Source: three-view drawing plus pictorial views. Frame: mm from the lowest corner of the part. A direction names the side the tool comes from. Coordinates: 2 decimals unless noted, no trailing zeros. Loops run counter-clockwise (first coordinate to the right, second up) from the corner with the lowest first, then second, coordinate; pieces in that order, holes last. Notation, with made-up numbers: M -2.75,83 L 10.25,83 A20 ccw 10.25,114 Z; hole C 43.5,-23 d9. An arc over 180 degrees is marked long. Use a Markdown table: item, result. Add a question column.
1. Set-up query: the marked faces 4 and 5. Return all of +Z, -Z, +X, -X, +Y, -Y with unobstructed straight access to the full face (end or side cutting, diameter ignored); none if empty.
2. Pin query (flat end, axial travel): pin 1 (4.5 mm diameter, centred on y = 13, z = 6.5, fed in from +X); pin 2 (3 mm diameter, centred on x = 29.95, y = 8, fed in from +Z); pin 3 (1.3 mm diameter, centred on y = 3, z = 8, fed in from +X). Return the tip coordinate at first contact, or that it passes through.
3. Section C-C on z = 20. Output: boundary loops of the cut face in (x, y).
4. Line query: L1, parallel to Y at x = 0.95, z = 7.5; L2, parallel to Z at x = 12, y = 10.75; L3, parallel to X at y = 9.75, z = 6.5. Output: solid intervals per line, ascending. Write a range as [from, to].
5. Draft query along Z for the marked faces 1, 2 and 3. Return one class per face: +Z half, -Z half, draft (parallel to the pull), parting line (faces both ways), or undercut.
6. Section B-B on y = 8. Output: boundary loops of the cut face in (x, z).
7. Section A-A on x = 6.5. Output: boundary loops of the cut face in (y, z).
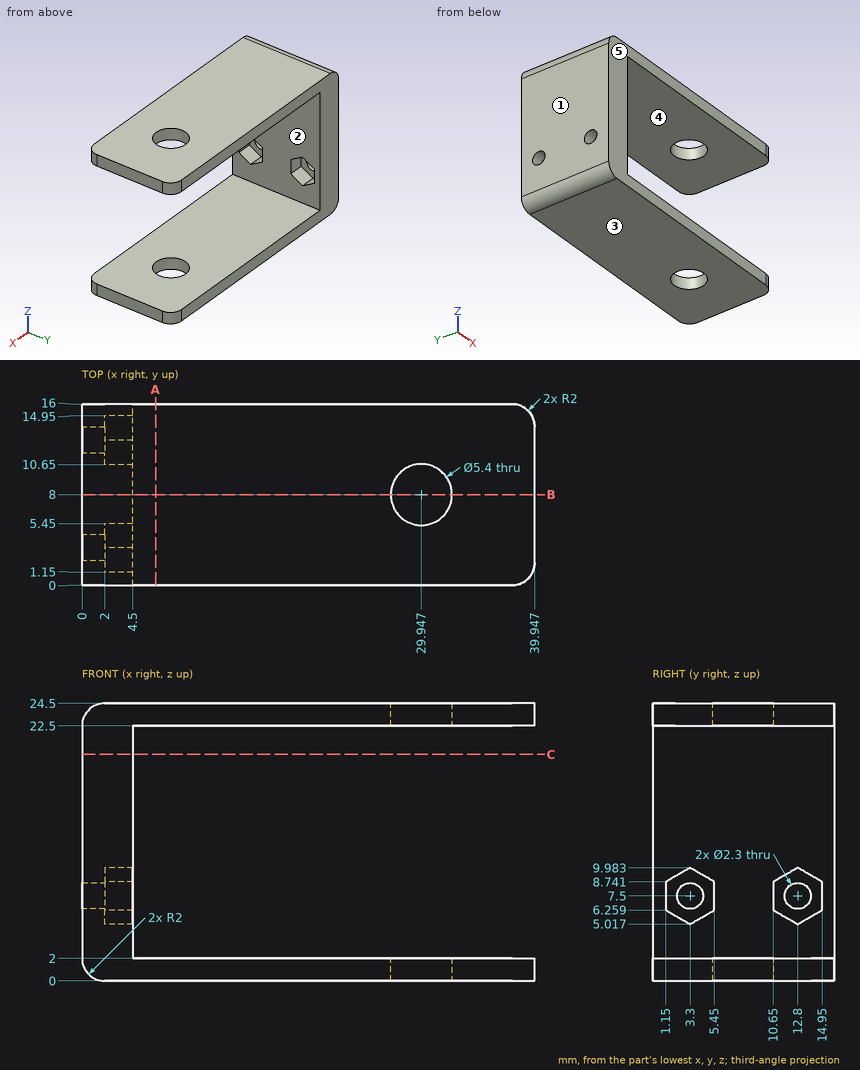
Answers below:
| question | item | result |
|---|---|---|
| 1 | face 4 | +X, +Y, -Y |
| 1 | face 5 | +Z, -Z, +X, -X, -Y |
| 2 | pin 1 | stops at x = 4.5 |
| 2 | pin 2 | passes through |
| 2 | pin 3 | stops at x = 2 |
| 3 | outline | M 0,0 L 4.5,0 L 4.5,16 L 0,16 Z |
| 4 | L1 | y = [0, 2.15], [4.45, 11.65], [13.95, 16] |
| 4 | L2 | z = [0, 2], [22.5, 24.5] |
| 4 | L3 | x = [0, 4.5] |
| 5 | face 1 | draft |
| 5 | face 2 | undercut |
| 5 | face 3 | -Z half |
| 6 | outline | M 0,2 A2 ccw 2,0 L 27.25,0 L 27.25,2 L 4.5,2 L 4.5,22.5 L 27.25,22.5 L 27.25,24.5 L 2,24.5 A2 ccw 0,22.5 Z; M 32.65,0 L 39.95,0 L 39.95,2 L 32.65,2 Z; M 32.65,22.5 L 39.95,22.5 L 39.95,24.5 L 32.65,24.5 Z |
| 7 | outline | M 0,0 L 16,0 L 16,2 L 0,2 Z; M 0,22.5 L 16,22.5 L 16,24.5 L 0,24.5 Z |
